```python
from build123d import *
from build123d.topology import SkipClean

# Parameters (mm, degrees)
STOCK_GOUX_START         = -74.233053816
STOCK_GOUX_LIKED_1_DEPTH = 57.798154544
BOSS_EXTRUDE1_DEPTH      = 57.798155
CUT_EXTRUDE1_DEPTH       = 117.763925236
SKETCH6_R                = 0.6
CUT_EXTRUDE2_DEPTH       = 156.868172362
CUT_EXTRUDE4_DEPTH       = 0.4


# Read off the part's stored shape, not the designer's step: Stock-Goux Liked-1
with BuildPart() as part:
    # Stock-Goux Liked-1 outline → Stock-Goux Liked-1 (new body)
    with BuildSketch(Plane(origin=(0, 0, 0), x_dir=(0.8164965809277323, 0.40824829046385713, 0.40824829046385636), z_dir=(0.5773502691896168, -0.5773502691896308, -0.5773502691896297)).offset(STOCK_GOUX_START)):
        Polygon((60.366452966, 115.851992166), (57.866453013, 120.182119103), (57.433440297, 119.932119095), (63.338140771, 109.704877872), (75.147541717, 109.704877872), (75.147541717, 110.204877888), (70.147541811, 110.204877888), (70.147541811, 113.704878), (65.647541921, 113.704878), (63.397541976, 117.601992222), align=None)
    extrude(amount=STOCK_GOUX_LIKED_1_DEPTH)

    # Sketch2 → Boss-Extrude1 (add)
    with SkipClean():  # the faces are left unmerged after this step: merging them gives an invalid solid
        with BuildSketch(Plane(origin=(-42.858473604, 42.858473604, 42.858473604), x_dir=(0.40824829046386124, -0.4082482904638709, 0.8164965809277231), z_dir=(-0.5773502691896168, 0.5773502691896305, 0.5773502691896301))):
            Polygon((132.580982015, -10.227241223), (123.723931305, -5.113620612), (126.676281542, 0), align=None)
        extrude(amount=-BOSS_EXTRUDE1_DEPTH)

    # Sketch5 → Cut-Extrude1 (cut, through all)
    with SkipClean():  # the faces are left unmerged after this step: merging them gives an invalid solid
        with BuildSketch(Plane(origin=(0, -80.401490288, 80.401490288), x_dir=(1, 0, 0), z_dir=(0, -0.7071067811865477, 0.7071067811865475))):
            Polygon((41.80289893, 54.586651387), (44.112300006, 51.320665064), (51.869017359, 56.805492503), (49.559616282, 60.071478827), align=None)
        cut_extrude1 = extrude(amount=-CUT_EXTRUDE1_DEPTH, mode=Mode.SUBTRACT)

    # Sketch6 → Cut-Extrude2 (cut, through all)
    with SkipClean():  # the faces are left unmerged after this step: merging them gives an invalid solid
        with BuildSketch(Plane(origin=(53.600993525, 26.800496763, 26.800496763), x_dir=(0.36514837167011016, 0.18257418583505447, -0.9128709291752772), z_dir=(0.8164965809277269, 0.4082482904638622, 0.40824829046386213))):
            with Locations(Location((-98.379129588, -56.52687032, 0), (0, 0, 90))):
                Circle(SKETCH6_R)
        cut_extrude2 = extrude(amount=-CUT_EXTRUDE2_DEPTH, mode=Mode.SUBTRACT)

    # Sketch8 → Cut-Extrude4 (cut)
    with SkipClean():  # the faces are left unmerged after this step: merging them gives an invalid solid
        with BuildSketch(Plane(origin=(0, -77.573063073, 77.573063073), x_dir=(1, 0, 0), z_dir=(0, 0.7071067811865477, -0.7071067811865475))):
            Polygon((32.655977778, -69.700657922), (32.580927697, -69.806236848), (28.99506031, -67.268526511), (28.554936111, -67.890551752), (28.062658467, -67.542014091), (28.502782665, -66.919988851), (27.305797489, -66.07281337), (27.670871608, -65.557639091), (28.867856784, -66.404814572), (30.608001015, -63.945970422), align=None)
            Polygon((29.360134428, -66.753352233), (31.50478587, -68.270890293), (30.431188114, -65.239630277), align=None, mode=Mode.SUBTRACT)
        extrude(amount=-CUT_EXTRUDE4_DEPTH, mode=Mode.SUBTRACT)

    # Mirror1: Cut-Extrude1, Cut-Extrude2 across plane
    with SkipClean():  # the faces are left unmerged after this step: merging them gives an invalid solid
        add(cut_extrude1.mirror(Plane(origin=(-26.173583561, 26.173583561, 26.173583561), x_dir=(0.40824829046388933, -0.4082482904638845, 0.8164965809277022), z_dir=(0.5773502691896123, -0.5773502691896054, -0.5773502691896596))), mode=Mode.SUBTRACT)
        add(cut_extrude2.mirror(Plane(origin=(-26.173583561, 26.173583561, 26.173583561), x_dir=(0.40824829046388933, -0.4082482904638845, 0.8164965809277022), z_dir=(0.5773502691896123, -0.5773502691896054, -0.5773502691896596))), mode=Mode.SUBTRACT)


solid = part.part
```
CAD build for the part. Positions are in the model's coordinates, mm. A direction names the side the tool comes from. Round coordinates to 2 decimals unless told otherwise and drop trailing zeros. Loops run counter-clockwise (first coordinate to the right, second up) from the corner with the lowest first, then second, coordinate; pieces in that order, holes last. Notation, with made-up numbers: M 10.25,-23 L 67.25,-23 A32 cw 67.25,16 Z; hole C 54,3 d9. An arc over 180 degrees is marked long. Use a Markdown table: item, result. Add a question column.
(1) Cut at A-A (y = -26). Give the cut face in (x, z).
(2) Cut at B-B (x = 20). Give the cut face in (y, z).
(3) Flat gauge pins, fed straight in: pin 1 (1.5 mm diameter, centred on x = 15, y = -15, fed in from -Z); pin 2 (12 mm diameter, centred on x = 12, y = -42.5, fed in from +Z); pin 3 (10 mm diameter, centred on y = -28, z = 132, fed in from -X); pin 4 (6 mm diameter, centred on x = 21, z = 140, fed in from +Y). Where does each tip first touch, or does it go through?
(4) Drill centre lines: line 1 (Y direction, x = 24, z = 141); line 2 (Y direction, x = 28, z = 140.5); line 3 (X direction, y = -26.5, z = 133.5). Where is each one in solid material? Low to high.
(5) Pull direction X, two halves, no side cores. Call faces 5 (the face through (30.976, -30.494, 124.931)), 6 (the face through (29.089, -26.295, 134.508)), 7 (the face through (20.49, -31.39, 131.09)), 8 (the face through (44.012, -39.304, 118.71)): +X half, -X half, draft (parallel to the pull), parting line (faces both ways), or undercut.
(6) Which spindle directions (+Z, -Z, +X, -X, +Y, -Y) get a long thin tool onto all of the face, cutting with end or side? Do faces 1 (the face through (21.875, -32.881, 133.978)), 2 (the face through (29.9, -31.05, 124.37)), 3 (the face through (26.288, -29.005, 134.515)), 4 (the face through (30.39, -29.96, 125.75)). Say none if no direction does.
Geometry says:
| question | item | result |
|---|---|---|
| 1 | outline | M 11.54,143.61 L 18.77,129.15 L 40.46,129.15 L 40.11,129.85 L 33.99,129.85 L 31.51,134.8 L 26,134.8 L 20.49,140.31 L 18.01,137.84 L 11.89,143.96 Z |
| 2 | outline | M -34.46,135.15 L -27.23,127.91 L -6.75,148.4 L -7.1,148.75 L -12.01,143.84 L -14.49,146.31 L -20,140.8 L -25.51,140.8 L -27.99,135.85 L -34.11,135.85 Z |
| 3 | pin 1 | stops at z = 139.4 |
| 3 | pin 2 | passes through |
| 3 | pin 3 | stops at x = 14.81 |
| 3 | pin 4 | stops at y = -12.15 |
| 4 | line 1 | y = -19.8 to -17.17, -14.85 to -14.15 |
| 4 | line 2 | y = -15.35 to -14.65 |
| 4 | line 3 | x = 16.84 to 32.41 |
| 5 | face 5 | undercut |
| 5 | face 6 | draft |
| 5 | face 7 | -X half |
| 5 | face 8 | +X half |
| 6 | face 1 | +Z, -Y |
| 6 | face 2 | -Z |
| 6 | face 3 | +Z, +X, -Y |
| 6 | face 4 | none |
